from build123d import *

# Parameters (mm, degrees)
SKETCH_1_W          = 83
SKETCH_1_H          = 53
SKETCH_1_W_2        = 80
SKETCH_1_H_2        = 50
EXTRUDE_1_DEPTH     = 1.2
SKETCH_1_4_W        = 3.5
SKETCH_1_4_H        = 3.5
EXTRUDE_2_DEPTH     = 19.8
EXTRUDE_3_DEPTH     = 1.2
SKETCH_3_W          = 20.8
SKETCH_3_H          = 1.4
EXTRUDE_4_DEPTH     = 15
SKETCH_4_W          = 12.8
SKETCH_4_H          = 1.4
EXTRUDE_5_DEPTH     = 5
SKETCH_5_W          = 28
SKETCH_5_H          = 17
CUT_EXTRUDE_1_DEPTH = 5
FILLET_2_R          = 1
FILLET_3_R          = 1
FILLET_4_R          = 1


with BuildPart() as part:
    # Sketch 1 → Extrude 1 (new body)
    with BuildSketch(Plane(origin=(0, 0, 0), x_dir=(1, 0, 0), z_dir=(0, 1, 0))):
        with Locations((40.1, 25.1)):
            Rectangle(SKETCH_1_W, SKETCH_1_H)
        with Locations((40, 25)):
            Rectangle(SKETCH_1_W_2, SKETCH_1_H_2, mode=Mode.SUBTRACT)
    extrude(amount=EXTRUDE_1_DEPTH)

    # Sketch 1_4 → Extrude 2 (add)
    with BuildSketch(Plane(origin=(0, 0, 0), x_dir=(1, 0, 0), z_dir=(0, 1, 0))):
        with Locations((1.75, 48.25)):
            Rectangle(SKETCH_1_4_W, SKETCH_1_4_H)
        with Locations((1.75, 1.75)):
            Rectangle(SKETCH_1_4_W, SKETCH_1_4_H)
        with Locations((78.25, 48.25)):
            Rectangle(SKETCH_1_4_W, SKETCH_1_4_H)
        with Locations((78.25, 1.75)):
            Rectangle(SKETCH_1_4_W, SKETCH_1_4_H)
    extrude(amount=EXTRUDE_2_DEPTH)

    # Sketch 1_5 → Extrude 3 (add)
    with BuildSketch(Plane(origin=(0, 0, 0), x_dir=(1, 0, 0), z_dir=(0, 1, 0))):
        Polygon((3.5, 3.5), (3.5, 0), (76.5, 0), (76.5, 3.5), (80, 3.5), (80, 46.5), (76.5, 46.5), (76.5, 50), (3.5, 50), (3.5, 46.5), (0, 46.5), (0, 3.5), align=None)
    extrude(amount=EXTRUDE_3_DEPTH)

    # Sketch 3 → Extrude 4 (add)
    with BuildSketch(Plane(origin=(0, 1.2, 0), x_dir=(1, 0, 0), z_dir=(0, 1, 0))):
        with Locations((15.3, 50.9)):
            Rectangle(SKETCH_3_W, SKETCH_3_H)
    extrude(amount=EXTRUDE_4_DEPTH)

    # Sketch 4 → Extrude 5 (add)
    with BuildSketch(Plane(origin=(0, 1.2, 0), x_dir=(1, 0, 0), z_dir=(0, 1, 0))):
        with Locations((40, -0.7)):
            Rectangle(SKETCH_4_W, SKETCH_4_H)
    extrude(amount=EXTRUDE_5_DEPTH)

    # Sketch 5 → Cut-Extrude 1 (cut)
    with BuildSketch(Plane(origin=(0, 1.2, 0), x_dir=(1, 0, 0), z_dir=(0, 1, 0))):
        with Locations((39.7, 38.1)):
            Rectangle(SKETCH_5_W, SKETCH_5_H)
    extrude(amount=-CUT_EXTRUDE_1_DEPTH, mode=Mode.SUBTRACT)

    # Fillet 2
    fillet_2_edges = [part.edges().sort_by_distance(p)[0] for p in [
        (25.7, 0.6, -29.6),
        (25.7, 0.6, -46.6),
        (53.7, 0.6, -46.6),
        (53.7, 0.6, -29.6),
        (-1.4, 0.6, 1.4),
        (-1.4, 0.6, -51.6),
        (81.6, 0.6, -51.6),
        (81.6, 0.6, 1.4),
    ]]
    fillet(fillet_2_edges, radius=FILLET_2_R)

    # Fillet 3
    fillet_3_edges = [part.edges().sort_by_distance(p)[0] for p in [
        (4.9, 16.2, -50.9),
        (25.7, 16.2, -50.9),
    ]]
    fillet(fillet_3_edges, radius=FILLET_3_R)

    # Fillet 4
    fillet_4_edges = [part.edges().sort_by_distance(p)[0] for p in [
        (33.6, 6.2, 0.7),
        (46.4, 6.2, 0.7),
    ]]
    fillet(fillet_4_edges, radius=FILLET_4_R)


solid = part.part
The listing builds one solid part. Answer for the finished solid, in the listing's coordinates (mm). A direction names the side the tool comes from. Coordinates: 2 decimals unless noted, no trailing zeros. Write each loop counter-clockwise with the first axis right and the second up, starting at its lowest first coordinate (ties: lowest second). Pieces come first, ordered by that corner, then holes. Notation, with made-up numbers: (57, 87) - (89, 87) arc R8 ccw to (89, 93) - close; hole circle Ø10 at (65.25, 11). An arc over 180 degrees is marked (long way). Answer as CSV lines item,"result".
1. Find section A-A (x = 42). Give the vertices of the cut face in (y, z).
Computed values:
outline,"(0, -51.6) - (1.2, -51.6) - (1.2, -46.6) - (0, -46.6) - close; (0, -29.6) - (1.2, -29.6) - (1.2, 0) - (6.2, 0) - (6.2, 1.4) - (0, 1.4) - close"
2. Find section D-D (z = -47.5). Give the vertices of the cut face in (x, y).
Computed values:
outline,"(-1.4, 0) - (81.6, 0) - (81.6, 1.2) - (80, 1.2) - (80, 19.8) - (76.5, 19.8) - (76.5, 1.2) - (3.5, 1.2) - (3.5, 19.8) - (0, 19.8) - (0, 1.2) - (-1.4, 1.2) - close"
3. Given P1, Ø1, axis at x = 2, y = 11.5, coming from the -Z side; P2, Ø3, axis at y = 10.5, z = -48.5, coming from the +X side; P3, Ø6, axis at x = 21, z = -21, coming from the +Y side; P4, Ø1.5, axis at y = 3.5, z = -20.5, coming from the +X side, each flat-ended and moving along its own axis, determine where each tip first touches the part or whether it passes through.
Computed values:
P1,"stops at z = -50"
P2,"stops at x = 80"
P3,"stops at y = 1.2"
P4,"passes through"
4. Determine the mould class of faces 6 (the flat face through (76.5, 10, -2)), 7 (the flat face through (80, 10, -48)), 8 (the flat face through (2, 19.8, -48)) for opening direction X: +X half, -X half, draft (parallel to the pull), parting line (faces both ways), or undercut.
Computed values:
face 6,"undercut"
face 7,"+X half"
face 8,"draft"
5. Find section B-B (y = 11.75). Give the vertices of the cut face in (x, z).
Computed values:
outline,"(0, -50) - (3.5, -50) - (3.5, -46.5) - (0, -46.5) - close; (0, -3.5) - (3.5, -3.5) - (3.5, 0) - (0, 0) - close; (4.9, -51.6) - (25.7, -51.6) - (25.7, -50.2) - (4.9, -50.2) - close; (76.5, -50) - (80, -50) - (80, -46.5) - (76.5, -46.5) - close; (76.5, -3.5) - (80, -3.5) - (80, 0) - (76.5, 0) - close"
6. Straight lines are drawn through the part: line 1 (X direction, y = 8, z = -49); line 2 (Y direction, x = 17.5, z = -36.5); line 3 (Z direction, x = 45, y = 3). For each, find the intervals that lie inside material, in ascending order. Write a range as [from, to].
Computed values:
line 1,"x = [0, 3.5], [76.5, 80]"
line 2,"y = [0, 1.2]"
line 3,"z = [0, 1.4]"
7. A tool of negligible diameter and unlimited length cuts with its end or side. For faces 1 (the flat face through (80, 10, -2)), 2 (the flat face through (2, 10, -3.5)), 3 (the flat face through (78, 10, -50)), 4 (the flat face through (15, 9, -50.2)), 5 (the flat face through (78, 10, 0)), from which of +Z, -Z, +X, -X, +Y, -Y can it reach the whole face along a straight path? Write none if from no direction.
Computed values:
face 1,"+Z, -Z, +X, +Y"
face 2,"+X, -X, +Y"
face 3,"-Z, +X, -X, +Y"
face 4,"+Z, +X, -X, +Y"
face 5,"+Z, +X, +Y"
8. Find section C-C (z = -42). Give the vertices of the cut face in (x, y), plus the area to 3 significant figures.
Computed values:
outline,"(-1.4, 0) - (25.7, 0) - (25.7, 1.2) - (-1.4, 1.2) - close; (53.7, 0) - (81.6, 0) - (81.6, 1.2) - (53.7, 1.2) - close"
area,"66.0 mm²"
